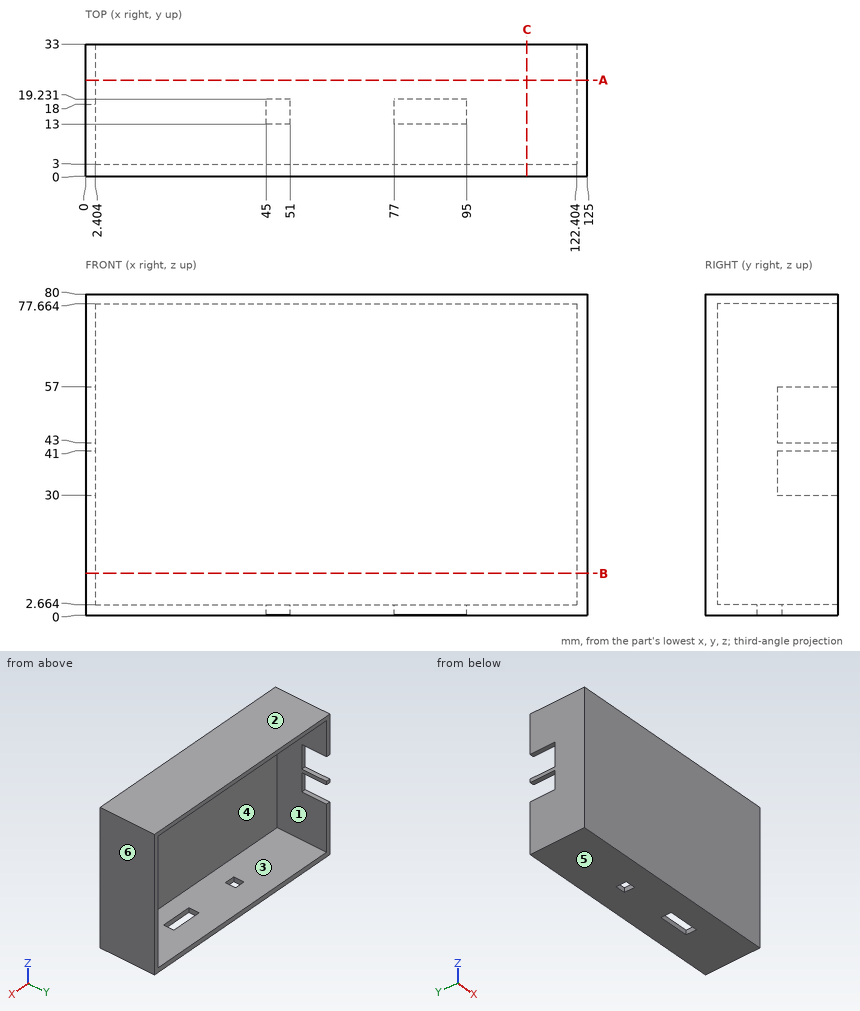
The drawing under review shows one solid part. Ordinate dimensions are in mm from its lowest x, y, z. A direction names the side the tool comes from. Give positions to 0.01 mm unless a question says otherwise; leave off trailing zeros. Write each loop counter-clockwise with the first axis right and the second up, starting at its lowest first coordinate (ties: lowest second). Pieces come first, ordered by that corner, then holes. Notation, with made-up numbers: M -7,21 L -1,21 A7 cw -1,28 Z; hole C -15,70.5 d2. An arc over 180 degrees is marked long. Write each question's results on one line, items separated by ' | '. Start each with the question number.
1. Insertion check: pin 1 Ø2.5 at (x, z) = (1, 50) entering from +Y; pin 2 Ø8 at (x, z) = (47.5, 35.5) entering from +Y. Each pin has a flat end and moves straight along its axis. Give the tip position at first contact, or say it passes through.
2. We need section B-B (z = 10.5). Write out the cut boundary in (x, y), and give its area (3 significant figures).
3. For probe 1 along Z at (x, y) = (48.5, 23.5); probe 2 along X at (y, z) = (10.5, 66.5); probe 3 along Y at (x, z) = (8, 5.5), list the stretches that pass through material, from the lowest coordinate up. Write a range as [from, to].
4. We need section A-A (y = 24). Write out the cut boundary in (x, z).
5. For the marked faces 1 and 2, list the 3-axis set-ups (+Z, -Z, +X, -X, +Y, -Y) from which the entire face can be reached by the end or side of a thin tool; tool diameter is ignored.
6. Mouldability with a two-part tool opening along X and no side actions: class the marked faces 3, 4, 5 and 6 as released by +X, released by -X, zero draft, split by the parting line, or undercut.
7. We need section C-C (x = 110). Write out the cut boundary in (y, z).
Results found:
1) pin 1: stops at y = 18 | pin 2: stops at y = 3
2) outline: M 0,0 L 125,0 L 125,33 L 122.4,33 L 122.4,3 L 2.4,3 L 2.4,33 L 0,33 Z | area: 525 mm^2
3) probe 1: z = [0, 2.66], [77.66, 80] | probe 2: x = [0, 2.4], [122.4, 125] | probe 3: y = [0, 3]
4) outline: M 0,0 L 125,0 L 125,80 L 0,80 L 0,57 L 2.4,57 L 2.4,77.66 L 122.4,77.66 L 122.4,2.66 L 2.4,2.66 L 2.4,30 L 0,30 Z; M 0,41 L 2.4,41 L 2.4,43 L 0,43 Z
5) face 1: +Y | face 2: +Z, +X, -X, +Y, -Y
6) face 3: undercut | face 4: undercut | face 5: zero draft | face 6: released by +X
7) outline: M 0,0 L 33,0 L 33,2.66 L 3,2.66 L 3,77.66 L 33,77.66 L 33,80 L 0,80 Z
